from build123d import *

# Parameters (mm, degrees)
F0_W     = 25.4
F0_H     = 25.4
F1_DEPTH = 25.4
F2_R     = 6.35
F3_DEPTH = 25.4
F4_R     = 6.35
F5_DEPTH = 76.2
F6_W     = 12.7
F6_H     = 12.7
F7_DEPTH = 76.2
F8_R     = 3.175
F9_DEPTH = 25.4


with BuildPart() as f1:
    # F0 (on Right) → F1 (new body)
    with BuildSketch(Plane.YZ):
        Rectangle(F0_W, F0_H)
    extrude(amount=F1_DEPTH)

    # F2 (on face) → F3 (cut)
    with BuildSketch(Plane.YZ.offset(25.4)):
        Circle(F2_R)
    extrude(amount=-F3_DEPTH, mode=Mode.SUBTRACT)

    # F4 (on face) → F5 (join)
    with BuildSketch(Plane.XY.offset(12.7)):
        with Locations((12.7, 0)):
            Circle(F4_R)
    extrude(amount=F5_DEPTH)

    # F6 (on face) → F7 (join)
    with BuildSketch(Plane(origin=(0, 12.7, 0), x_dir=(-1, 0, 0), z_dir=(0, 1, 0))):
        with Locations((-12.7, 0)):
            Rectangle(F6_W, F6_H)
    extrude(amount=F7_DEPTH)

    # F8 (on face) → F9 (cut)
    with BuildSketch(Plane(origin=(6.35, 0, 0), x_dir=(0, -1, 0), z_dir=(-1, 0, 0))):
        with Locations((-79.375, 0)):
            Circle(F8_R)
    extrude(amount=-F9_DEPTH, mode=Mode.SUBTRACT)


solid = f1.part
CAD build for the part. Positions are in the model's coordinates, mm. A direction names the side the tool comes from. Round coordinates to 2 decimals unless told otherwise and drop trailing zeros. Write each loop counter-clockwise with the first axis right and the second up, starting at its lowest first coordinate (ties: lowest second). Pieces come first, ordered by that corner, then holes. Notation, with made-up numbers: (52.25, 59) -> (66.25, 59) arc R33 ccw to (66.25, 97) -> close; hole circle Ø1 at (87.25, -27). An arc over 180 degrees is marked (long way). Answer as a JSON object with one key per item and string values.
(1) Two-plate mould, pull along Z, no slides. Class faces 1 (the face through (13, 50, -6.35)), 2 (the face through (13, -12.7, 0)), 3 (the face through (12.611, 76.347, 0.954)): +Z half, -Z half, draft (parallel to the pull), parting line (faces both ways), or undercut.
Reported:
{"face 1": "-Z half", "face 2": "draft", "face 3": "undercut"}
(2) Band-saw the part on D-D, the plane z = 42. List the corners of the cut face in (x, y), then the cut area to 3 significant figures.
Reported:
{"outline": "circle Ø12.7 at (12.7, 0)", "area": "127 mm^2"}
(3) Band-saw the part on C-C, the plane x = 12.7. List the corners of the cut face in (y, z) (3 decimals).
Reported:
{"outline": "(-12.7, -12.7) -> (12.7, -12.7) -> (12.7, -6.35) -> (88.9, -6.35) -> (88.9, 6.35) -> (12.7, 6.35) -> (12.7, 12.7) -> (6.35, 12.7) -> (6.35, 88.9) -> (-6.35, 88.9) -> (-6.35, 12.7) -> (-12.7, 12.7) -> close; hole circle Ø12.7 at (0, 0); hole circle Ø6.35 at (79.375, 0)"}
(4) Which spindle directions (+Z, -Z, +X, -X, +Y, -Y) get a long thin tool onto all of the face, cutting with end or side? Do faces 4 (the face through (6.35, 50, 0)), 5 (the face through (19.05, 50, 0)), 6 (the face through (13, 50, 6.35)). Say none if no direction does.
Reported:
{"face 4": "+Z, -Z, -X, +Y", "face 5": "+Z, -Z, +X, +Y", "face 6": "+Z, +X, -X, +Y"}
(5) Band-saw the part on B-B, the plane y = 0. List the corners of the cut face in (x, z).
Reported:
{"outline": "(0, -12.7) -> (25.4, -12.7) -> (25.4, -6.35) -> (0, -6.35) -> close; (0, 6.35) -> (25.4, 6.35) -> (25.4, 12.7) -> (19.05, 12.7) -> (19.05, 88.9) -> (6.35, 88.9) -> (6.35, 12.7) -> (0, 12.7) -> close"}
(6) Band-saw the part on A-A, the plane z = 0. List the corners of the cut face in (x, y), then the cut area to 3 significant figures.
Reported:
{"outline": "(0, -12.7) -> (25.4, -12.7) -> (25.4, -6.35) -> (0, -6.35) -> close; (0, 6.35) -> (25.4, 6.35) -> (25.4, 12.7) -> (19.05, 12.7) -> (19.05, 76.2) -> (6.35, 76.2) -> (6.35, 12.7) -> (0, 12.7) -> close; (6.35, 82.55) -> (19.05, 82.55) -> (19.05, 88.9) -> (6.35, 88.9) -> close", "area": "1,210 mm^2"}
(7) Pin check, flat tips, straight feed: P1, Ø12.5, axis at x = 7.5, y = -6, coming from the +Z side; P2, Ø12, axis at x = 18.5, y = 68, coming from the +Z side; P3, Ø4, axis at x = 11.5, y = 62.5, coming from the -Z side; P4, Ø1.5, axis at x = 9.5, z = 45, coming from the -Y side. Stop position of each tip, or through.
Reported:
{"P1": "stops at z = 88.9", "P2": "stops at z = 6.35", "P3": "stops at z = -6.35", "P4": "stops at y = -5.86"}
(8) Probe probe 1 along Z at (x, y) = (17.25, 0); probe 2 along Z at (x, y) = (16.5, 71); probe 3 along Z at (x, y) = (13.5, 10). List the from-to ranges inside material, lowest first. Write a range as [from, to].
Reported:
{"probe 1": "z = [-12.7, -6.35], [6.35, 88.9]", "probe 2": "z = [-6.35, 6.35]", "probe 3": "z = [-12.7, 12.7]"}
